Source: three-view drawing plus pictorial views. Frame: mm from the lowest corner of the part. A direction names the side the tool comes from. Give positions to 0.01 mm unless a question says otherwise; leave off trailing zeros. Order: outer loops, then holes, each group sorted by start corner. A loop starts at its lowest first (then second) coordinate and runs counter-clockwise, first axis right, second up. Notation, with made-up numbers: (80.25, 89) - (90.25, 89) arc R18 cw to (90.25, 120) - close; hole circle Ø7 at (-8, 27.5). An arc over 180 degrees is marked (long way). Answer in a Markdown table with one row per item. Add a question column.
1. Section query B-B on z = 2.95. Return loops of the section in (x, y).
2. Contact query for a flat-ended pin moving along its axis: pin 1 (1 mm diameter, centred on x = 35.5, y = 6.5, fed in from +Z). Output: stop coordinate, or through.
3. Section query D-D on y = 9.25. Return loops of the section in (x, z).
4. Ray query, line 1 (Y direction, x = 29.5, z = 0.3) (1 decimal); line 2 (X direction, y = 8.5, z = 0.5); line 3 (X direction, y = 2, z = 4.45). Return the intervals inside material, ascending. Write a range as [from, to].
5. Access query for the marked faces 1 and 2. Directions: +Z, -Z, +X, -X, +Y, -Y. A direction counts if a zero-diameter tool reaches every point of the face in a straight line with its end or side. Return the directions, or none.
6. Section query C-C on y = 4.25. Return loops of the section in (x, z).
7. Section query A-A on x = 29.5. Return loops of the section in (y, z) (1 decimal).
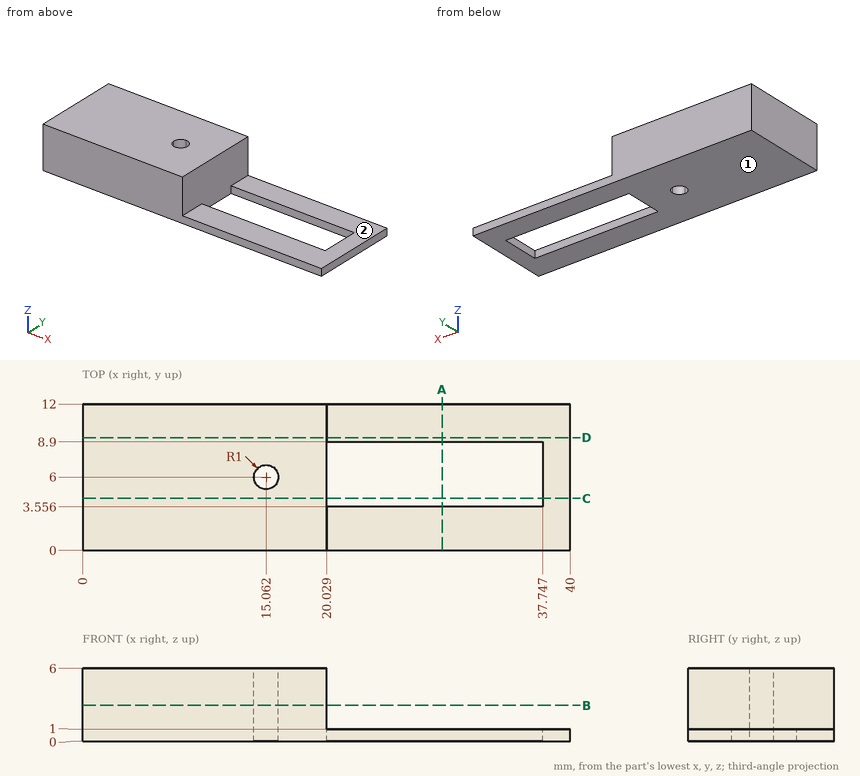
Answer:
| question | item | result |
|---|---|---|
| 1 | outline | (0, 0) - (20.03, 0) - (20.03, 12) - (0, 12) - close; hole circle Ø2 at (15.06, 6) |
| 2 | pin 1 | passes through |
| 3 | outline | (0, 0) - (40, 0) - (40, 1) - (20.03, 1) - (20.03, 6) - (0, 6) - close |
| 4 | line 1 | y = [0, 3.6], [8.9, 12] |
| 4 | line 2 | x = [0, 20.03], [37.75, 40] |
| 4 | line 3 | x = [0, 20.03] |
| 5 | face 1 | -Z, +X, -X, +Y, -Y |
| 5 | face 2 | +Z, +X, +Y, -Y |
| 6 | outline | (0, 0) - (20.03, 0) - (20.03, 6) - (0, 6) - close; (37.75, 0) - (40, 0) - (40, 1) - (37.75, 1) - close |
| 7 | outline | (0, 0) - (3.6, 0) - (3.6, 1) - (0, 1) - close; (8.9, 0) - (12, 0) - (12, 1) - (8.9, 1) - close |
